from build123d import *

# Parameters (mm, degrees)
F2_SIZE  = 1
F4_R     = 3
F5_DEPTH = 39.4


with BuildPart() as f1:
    # F0 (on Front) → F1 (revolve)
    with BuildSketch(Plane.XZ):
        Polygon((-103.14801, 10), (-103.14801, 0), (166.85199, 0), (166.85199, 5), (154.85199, 5), (154.85199, 4), (153.35199, 4), (153.35199, 6), (-93.14801, 6), (-93.14801, 10), align=None)
    revolve(axis=Axis((31.85199, 0, 0), (1, 0, 0)))

    # F2
    f2_edges = [f1.edges().sort_by_distance(p)[0] for p in [
        (153.35199, 0, -6),
        (-103.14801, 0, -10),
        (166.85199, 0, -5),
    ]]
    chamfer(f2_edges, length=F2_SIZE)

    # F4 (on offset) → F5 (cut)
    with BuildSketch(Plane.XZ.offset(25)):
        with Locations((-97.64801, 0)):
            Circle(F4_R)
    extrude(amount=-F5_DEPTH, mode=Mode.SUBTRACT)


solid = f1.part
Work out the finished part from the listing and answer in its coordinate system (mm). A direction names the side the tool comes from. Coordinates: 2 decimals unless noted, no trailing zeros. Loops run counter-clockwise (first coordinate to the right, second up) from the corner with the lowest first, then second, coordinate; pieces in that order, holes last. Notation, with made-up numbers: (-23.5, 34.5) -> (-18.5, 34.5) arc R26 ccw to (-18.5, 57.5) -> close; hole circle Ø9 at (-35.5, 58.25). An arc over 180 degrees is marked (long way). Write each question's results on one line, items separated by ' | '. Start each with the question number.
1) Find section A-A on y = 0. Determine the outline of the cut face in (x, z), then the cut area to 3 significant figures.
2) For faces 1 (the cylindrical face through (28, 0, -6)), 2 (the flat face through (-103.148, 0, 0)), 3 (the cylindrical face through (154.091, 3.905, -0.867)), determine the directions among +Z, -Z, +X, -X, +Y, -Y from which every point of the face is accessible in a straight line to the end or side of a thin tool.
3) The mould has two halves that part along X. Classify faces 4 (the flat face through (-93.148, 0, -7)), 5 (the cylindrical face through (-94.787, -0.14, 0.901)), 6 (the cylindrical face through (160.27, 4.88, -1.08)): pulls with the +X half, pulls with the -X half, needs draft (parallel to the pull), parting line crosses it, or undercut.
4) Consider line 1 along X through (y, z) = (-0.25, 0); line 2 along X through (y, z) = (-4.75, 0); line 3 along X through (y, z) = (8.25, 0). Determine where each line is inside the solid, lowest interval first.
5) Find section B-B on x = -24. Determine the outline of the cut face in (y, z), then the cut area to 3 significant figures.
6) Flat-ended cylindrical pins translate along their axes: P1, Ø1.5, axis at x = 16, z = -2.5, coming from the +Y side; P2, Ø1.5, axis at x = 92.5, z = -6, coming from the +Y side; P3, Ø6, axis at x = 27, z = -4, coming from the +Y side; P4, Ø9.5, axis at x = -97.65, z = 0, coming from the -Y side. Find the tip coordinate at first contact, or state that the pin passes through.
Response values:
1) outline: (-103.15, -9) -> (-102.15, -10) -> (-93.15, -10) -> (-93.15, -6) -> (152.35, -6) -> (153.35, -5) -> (153.35, -4) -> (154.85, -4) -> (154.85, -5) -> (165.85, -5) -> (166.85, -4) -> (166.85, 4) -> (165.85, 5) -> (154.85, 5) -> (154.85, 4) -> (153.35, 4) -> (153.35, 5) -> (152.35, 6) -> (-93.15, 6) -> (-93.15, 10) -> (-102.15, 10) -> (-103.15, 9) -> close; hole circle Ø6 at (-97.65, 0) | area: 3,260 mm^2
2) face 1: +X | face 2: +Z, -Z, -X, +Y, -Y | face 3: none
3) face 4: pulls with the +X half | face 5: undercut | face 6: needs draft
4) line 1: x = -103.15 to -100.65, -94.65 to 166.85 | line 2: x = -103.15 to -100.65, -94.65 to 153.35, 154.85 to 166.1 | line 3: x = -103.15 to -100.65, -94.65 to -93.15
5) outline: circle Ø12 at (0, 0) | area: 113 mm^2
6) P1: stops at y = 5.74 | P2: stops at y = 2.9 | P3: stops at y = 5.92 | P4: stops at y = -10
